Can you work these out from the model? Positions are in its coordinate system, mm. Face numbers are marked on the shaded views. A direction names the side the tool comes from. Give positions to 0.01 mm unless a question says otherwise; leave off trailing zeros. Order: outer loops, then holes, each group sorted by start corner. A loop starts at its lowest first (then second) coordinate and runs counter-clockwise, first axis right, second up. Notation, with made-up numbers: M 44.5,-33 L 68.5,-33 A28 cw 68.5,-12 Z; hole C -10,-17 d7. An arc over 180 degrees is marked long. One line per question, with ' | ' between items. Start each with the question number.
1) For the marked faces 1 and 2, which set-ups out of +Z, -Z, +X, -X, +Y, -Y let a thin tool reach every point of the face, with its end or its side?
2) If we section it at B-B, the plane z = -2.5: Please give me the cut outline in (x, y).
3) If we section it at A-A, the plane y = 45.5: Please give me the cut outline in (x, z).
4) I'm going to push flat-ended pins straight in: pin 1 Ø2 at (x, y) = (-52.5, 43) entering from +Z; pin 2 Ø1.5 at (x, z) = (7, -26.5) entering from -Y; pin 3 Ø3.5 at (x, z) = (-3, -26.5) entering from +Y. Where does each tip first touch, or does it pass through?
5) Thinking about a two-plate mould opening in Y: for the marked faces 3, 4, 5 and 6, which applies, +Y half, -Y half, draft (parallel to the pull), parting line (faces both ways), or undercut?
6) Please list where these lines run through material, in increasing order: line 1 along Y through (x, z) = (-28, 5); line 2 along Y through (x, z) = (-63.5, 41); line 3 along Y through (x, z) = (0.5, 24). Write a range as [from, to].
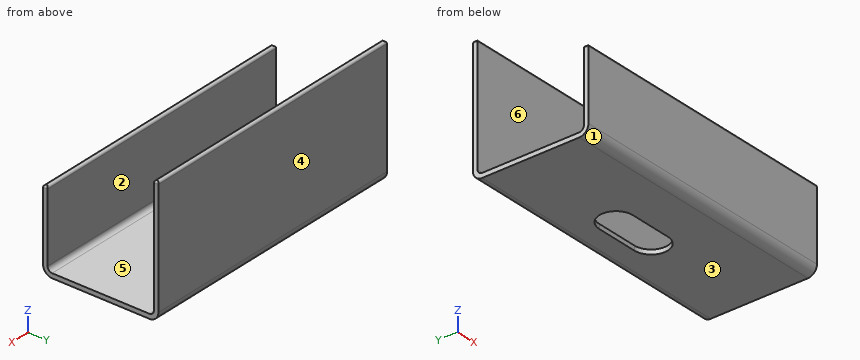
```python
from build123d import *

# Parameters (mm, degrees)
SKETCH1_W           = 183
SKETCH1_H           = 50
BOSS_EXTRUDE1_DEPTH = 3
SKETCH2_W           = 183
SKETCH2_H           = 76
BOSS_EXTRUDE2_DEPTH = 3
SKETCH3_W           = 183
SKETCH3_H           = 3
BOSS_EXTRUDE3_DEPTH = 80
FILLET2_R           = 1.5
CUT_EXTRUDE1_REACH  = 145.347
FILLET3_R           = 3
FILLET4_R           = 6


with BuildPart() as part:
    # Sketch1 → Boss-Extrude1 (new body)
    with BuildSketch(Plane(origin=(0, 0, 0), x_dir=(1, 0, 0), z_dir=(0, 1, 0))):
        Rectangle(SKETCH1_W, SKETCH1_H)
    extrude(amount=BOSS_EXTRUDE1_DEPTH)

    # Sketch2 → Boss-Extrude2 (add)
    with BuildSketch(Plane(origin=(0, 0, -25), x_dir=(-1, 0, 0), z_dir=(0, 0, -1))):
        with Locations((0, 38)):
            Rectangle(SKETCH2_W, SKETCH2_H)
    extrude(amount=BOSS_EXTRUDE2_DEPTH)

    # Sketch3 → Boss-Extrude3 (add)
    with BuildSketch(Plane.XY.offset(-25)):
        with Locations((0, 74.5)):
            Rectangle(SKETCH3_W, SKETCH3_H)
    extrude(amount=BOSS_EXTRUDE3_DEPTH)

    # Fillet2
    fillet2_edges = [part.edges().sort_by_distance(p)[0] for p in [
        (0, 3, 25),
        (-91.5, 74.5, 55),
        (0, 73, 55),
        (91.5, 74.5, 55),
        (0, 76, 55),
        (0, 0, 25),
        (91.5, 1.5, 25),
        (-91.5, 1.5, 25),
    ]]
    fillet(fillet2_edges, radius=FILLET2_R - 0.0001)  # a hair under: the kernel refuses the full size

    # Sketch4 → Cut-Extrude1 (cut, up to next)
    with BuildSketch(Plane.XY.offset(-25), mode=Mode.PRIVATE) as cut_extrude1_sk1:
        with BuildLine():
            Line((-14, 56.5), (14, 56.5))
            ThreePointArc((14, 56.5), (25, 45.5), (14, 34.5))
            Line((14, 34.5), (-14, 34.5))
            ThreePointArc((-14, 34.5), (-25, 45.5), (-14, 56.5))
        make_face()
    cut_extrude1_tool1 = extrude(cut_extrude1_sk1.sketch, amount=-CUT_EXTRUDE1_REACH, mode=Mode.PRIVATE) & part.part
    add(cut_extrude1_tool1.solids().sort_by_distance((0, 45.5, -25))[0], mode=Mode.SUBTRACT)

    # Fillet3
    fillet3_edges = [part.edges().sort_by_distance(p)[0] for p in [
        (0, 73, -25),
        (0, 3, -25),
    ]]
    fillet(fillet3_edges, radius=FILLET3_R)

    # Fillet4
    fillet4_edges = [part.edges().sort_by_distance(p)[0] for p in [
        (0, 0, -28),
        (0, 76, -28),
    ]]
    fillet(fillet4_edges, radius=FILLET4_R)


solid = part.part
```
Results found:
1) face 1: -Z, +X, -X, -Y | face 2: +Z, +X, -X
2) outline: M -91.5,0 L 91.5,0 L 91.5,3 L -91.5,3 Z; M -91.5,73 L 91.5,73 L 91.5,76 L -91.5,76 Z
3) outline: M -91.5,-28 L -25,-28 L -25,-25 L -91.5,-25 Z; M 25,-28 L 91.5,-28 L 91.5,-25 L 25,-25 Z
4) pin 1: stops at z = -25 | pin 2: stops at y = 1.32 | pin 3: stops at y = 75.33
5) face 3: draft | face 4: +Y half | face 5: undercut | face 6: undercut
6) line 1: y = [0, 3], [73, 76] | line 2: y = [73, 76] | line 3: y = [0.09, 2.91], [73, 76]
